Here's the drawing with two shaded views (mm, measured from the low corner). I have some questions. Round coordinates to 2 decimals unless told otherwise and drop trailing zeros. Order: outer loops, then holes, each group sorted by start corner. A loop starts at its lowest first (then second) coordinate and runs counter-clockwise, first axis right, second up. Notation, with made-up numbers: (-24, 12) -> (28, 12) arc R9 cw to (28, 16) -> close; hole circle Ø9 at (-22.75, 9.5). An arc over 180 degrees is marked (long way). Use a Markdown table: item, result. Add a question column.
Q1. If we section it at C-C on z = 0.65: Give the number of separate pieces and of enclosed holes in the cut face, plus the area to 3 significant figures.
Q2. If we section it at A-A on x = 32: List the corners of the cut face in (y, z) for me.
Q3. I need wall thicknesses on line 1 along Y through (x, z) = (2, 2.25); line 2 along X through (y, z) = (51, 2.4); line 3 along X through (y, z) = (12.5, 0.2) (1 decimal). Which ranges of each line are inside material? Lowest first, please. Write a range as [from, to].
Q4. If we section it at D-D on x = 21.5: List the corners of the cut face in (y, z) for me.
Q5. If we section it at B-B on y = 12.8: List the corners of the cut face in (x, z) for me.
Q6. I'm going to push flat-ended pins straight in: pin 1 Ø1.5 at (y, z) = (35, 1.5) entering from -X; pin 2 Ø0.9 at (x, z) = (44, 1) entering from +Y; pin 3 Ø1.5 at (y, z) = (32, 1.5) entering from +X; pin 4 Ø1.5 at (x, z) = (2, 1.5) entering from -Y. Where does each tip first touch, or does it pass through?
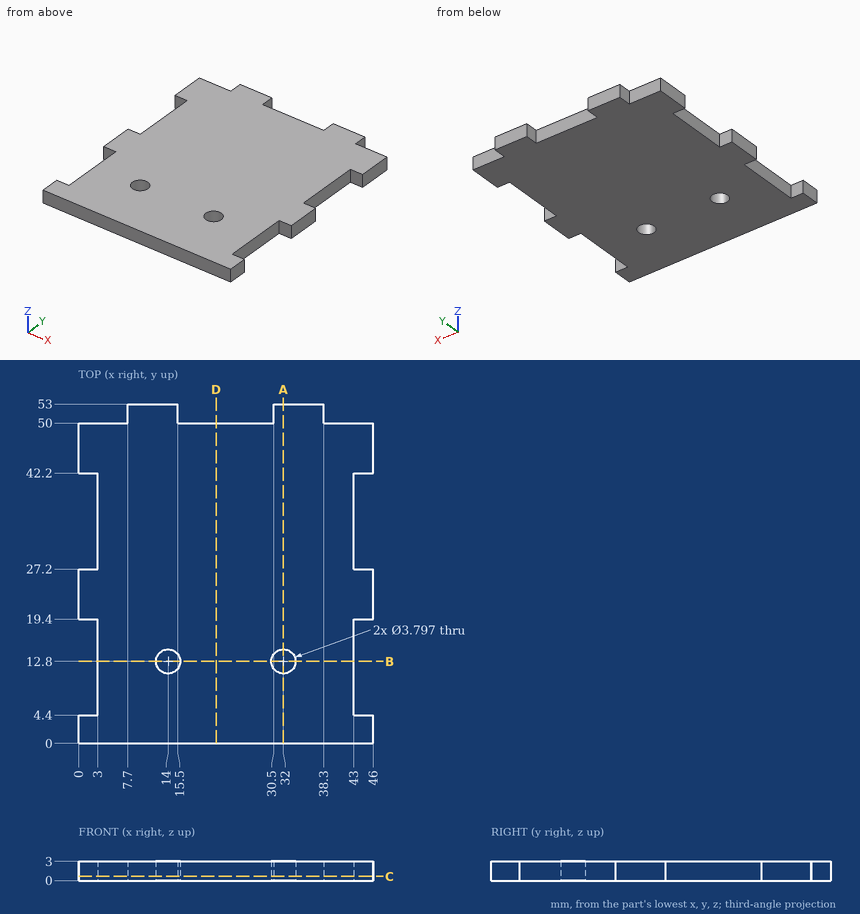
Answer below:
| question | item | result |
|---|---|---|
| 1 | separate pieces | 1 |
| 1 | enclosed holes | 2 |
| 1 | area | 2,140 mm² |
| 2 | outline | (0, 0) -> (10.9, 0) -> (10.9, 3) -> (0, 3) -> close; (14.7, 0) -> (53, 0) -> (53, 3) -> (14.7, 3) -> close |
| 3 | line 1 | [0, 4.4], [19.4, 27.2], [42.2, 50] |
| 3 | line 2 | [7.7, 15.5], [30.5, 38.3] |
| 3 | line 3 | [3, 12.1], [15.9, 30.1], [33.9, 43] |
| 4 | outline | (0, 0) -> (50, 0) -> (50, 3) -> (0, 3) -> close |
| 5 | outline | (3, 0) -> (12.1, 0) -> (12.1, 3) -> (3, 3) -> close; (15.9, 0) -> (30.1, 0) -> (30.1, 3) -> (15.9, 3) -> close; (33.9, 0) -> (43, 0) -> (43, 3) -> (33.9, 3) -> close |
| 6 | pin 1 | x = 3 |
| 6 | pin 2 | y = 50 |
| 6 | pin 3 | x = 43 |
| 6 | pin 4 | y = 0 |
